```python
from build123d import *

# Parameters (mm, degrees)
SKETCH1_R           = 11.9
SKETCH1_W           = 2.4
SKETCH1_H           = 5
BOSS_EXTRUDE2_DEPTH = 2
SKETCH2_W           = 2.3
SKETCH2_H           = 2.4
BOSS_EXTRUDE3_DEPTH = 4.7
SKETCH4_W           = 2.3
SKETCH4_H           = 2.3
BOSS_EXTRUDE5_DEPTH = 1.2
SKETCH5_W           = 2.3
SKETCH5_H           = 2.3
BOSS_EXTRUDE6_DEPTH = 1.2


with BuildPart() as part:
    # Sketch1 → Boss-Extrude2 (new body)
    with BuildSketch(Plane.XY):
        Circle(SKETCH1_R)
        with Locations((10, 0)):
            Rectangle(SKETCH1_W, SKETCH1_H, mode=Mode.SUBTRACT)
    extrude(amount=BOSS_EXTRUDE2_DEPTH)

    # Sketch2 → Boss-Extrude3 (add)
    with BuildSketch(Plane.XY.offset(2)):
        with Locations((-10, 0)):
            Rectangle(SKETCH2_W, SKETCH2_H)
    extrude(amount=BOSS_EXTRUDE3_DEPTH)

    # Sketch4 → Boss-Extrude5 (add)
    with BuildSketch(Plane(origin=(0, 1.2, 0), x_dir=(1, 0, 0), z_dir=(0, 1, 0))):
        with Locations((-10, -5.55)):
            Rectangle(SKETCH4_W, SKETCH4_H)
    extrude(amount=BOSS_EXTRUDE5_DEPTH)

    # Sketch5 → Boss-Extrude6 (add)
    with BuildSketch(Plane.XZ.offset(1.2)):
        with Locations((-10, 5.55)):
            Rectangle(SKETCH5_W, SKETCH5_H)
    extrude(amount=BOSS_EXTRUDE6_DEPTH)


solid = part.part
```
Model file for the job. Use its own axes, mm. A direction names the side the tool comes from. Coordinates: 2 decimals unless noted, no trailing zeros. Order: outer loops, then holes, each group sorted by start corner. A loop starts at its lowest first (then second) coordinate and runs counter-clockwise, first axis right, second up. Notation, with made-up numbers: (63, 89) -> (70, 89) arc R8 ccw to (70, 102) -> close; hole circle Ø11 at (49.5, 10.25). An arc over 180 degrees is marked (long way). Return JSON: item names as keys, results as strings.
Item 1: Mould opens along X. For faces 1 (the face through (8.8, 0, 1)), 2 (the face through (10, -2.5, 1)), 3 (the face through (-11.15, 0, 5)), 4 (the face through (-10, 2.4, 6)) say: pulls with the +X half, pulls with the -X half, needs draft (parallel to the pull), parting line crosses it, or undercut.
Model answer:
{"face 1": "undercut", "face 2": "undercut", "face 3": "pulls with the -X half", "face 4": "needs draft"}
Item 2: Slice it at C-C (x = 0). Write the cut outline in (y, z).
Model answer:
{"outline": "(-11.9, 0) -> (11.9, 0) -> (11.9, 2) -> (-11.9, 2) -> close"}
Item 3: Pin check, flat tips, straight feed: P1, Ø2.5, axis at x = -10.5, z = 5.5, coming from the +Y side; P2, Ø1, axis at x = -8, z = 1, coming from the -Y side; P3, Ø4, axis at x = 3, z = 2, coming from the +Y side. Stop position of each tip, or through.
Model answer:
{"P1": "stops at y = 2.4", "P2": "stops at y = -9.24", "P3": "stops at y = 11.86"}
Item 4: Slice it at B-B (x = 9.5). Write the cut outline in (y, z), then the cut area to 3 significant figures.
Model answer:
{"outline": "(-7.17, 0) -> (-2.5, 0) -> (-2.5, 2) -> (-7.17, 2) -> close; (2.5, 0) -> (7.17, 0) -> (7.17, 2) -> (2.5, 2) -> close", "area": "18.7 mm²"}
Item 5: Wall check: line 1 along X through (y, z) = (-2, 5.5); line 2 along Y through (x, z) = (0, 0.5); line 3 along Z through (x, y) = (-7, 2.75). Give the ranges that are in metal, low to high. Write a range as from..to.
Model answer:
{"line 1": "x = -11.15..-8.85", "line 2": "y = -11.9..11.9", "line 3": "z = 0..2"}
Item 6: Slice it at D-D (y = -10.5). Write the cut outline in (x, z).
Model answer:
{"outline": "(-5.6, 0) -> (5.6, 0) -> (5.6, 2) -> (-5.6, 2) -> close"}
Item 7: 3-axis set-ups, long thin cutter, end or side, ignore diameter. For faces 5 (the face through (-8.85, 0, 5)), 6 (the face through (-10, 1.2, 3)), 7 (the face through (-10, -2.4, 6)), 8 (the face through (10, 2.5, 1)): which of +Z, -Z, +X, -X, +Y, -Y reach the whole face in a straight line?
Model answer:
{"face 5": "+Z, +X, +Y, -Y", "face 6": "+X, -X, +Y", "face 7": "+Z, +X, -X, -Y", "face 8": "+Z, -Z"}
Item 8: Slice it at A-A (y = 0). Write the cut outline in (x, z), then the cut area to 3 significant figures.
Model answer:
{"outline": "(-11.9, 0) -> (8.8, 0) -> (8.8, 2) -> (-8.85, 2) -> (-8.85, 6.7) -> (-11.15, 6.7) -> (-11.15, 2) -> (-11.9, 2) -> close; (11.2, 0) -> (11.9, 0) -> (11.9, 2) -> (11.2, 2) -> close", "area": "53.6 mm²"}
